Autodesk Fusion 360 part; units mm, degrees
sketch "Sketch1" plane through (0, 0, 0) normal (0, 0, 1) x (1, 0, 0)
  circle A0 centre (0, 0) radius 10.1
  dimension "d1" = 20.2
extrude "Extrude1" add sketch "Sketch1" along normal blind 13.95
sketch "Sketch2" plane through (0, 0, 13.95) normal (0, 0, 1) x (-1, 0, 0)
  circle A0 centre (0, 0) radius 10.1
  circle A1 centre (0, 0) radius 17.5
  line L0 (-27.5, -17.6099) -> (27.5, -17.6099)
  line L1 (27.5, -17.6099) -> (27.5, 17.6099)
  line L2 (27.5, 17.6099) -> (-27.5, 17.6099)
  line L3 (-27.5, 17.6099) -> (-27.5, -17.6099)
  line L4 (-27.5, -17.6099) -> (27.5, 17.6099) construction
  line L5 (27.5, -17.6099) -> (-27.5, 17.6099) construction
  line L6 (-27.5, -17.6099) -> (-42.678, -17.6099)
  line L7 (-42.678, -17.6099) -> (-42.678, 17.6539)
  line L8 (-42.678, 17.6539) -> (-27.5, 17.6539)
  line L9 (-27.5, 17.6539) -> (-27.5, -17.6099)
  dimension "d4" = 35
  dimension "d7" = 55
extrude "Extrude2" add sketch "Sketch2" along normal blind 2 contours A0 | A1
extrude "Extrude3" add sketch "Sketch2" along normal blind 2 contours L0 L1 L2 L3 L9
sketch "Sketch3" plane through (0, 0, 13.95) normal (0, 0, 1) x (-1, 0, 0)
  circle A0 centre (11.0543, 10.2607) radius 1.5
  dimension "d10" = 3
extrude "Extrude4" add sketch "Sketch2" along normal blind 2 contours L3 L6 L7 L8 L9
sketch "Sketch5" plane through (0, -17.6099, 0) normal (0, -1, 0) x (1, 0, 0)
  line L0 (-27.5, 13.95) -> (27.5, 13.95)
  line L1 (27.5, 13.95) -> (27.5, 15.95)
  line L2 (27.5, 15.95) -> (-27.5, 15.95)
  line L3 (-27.5, 15.95) -> (-27.5, 13.95)
  line L4 (-27.5, 15.95) -> (42.6781, 15.95)
  line L5 (42.6781, 15.95) -> (42.6781, 13.95)
  line L6 (42.6781, 13.95) -> (-27.5, 13.95)
  line L7 (-27.5, 13.95) -> (-27.5, 15.95)
extrude "Extrude5" add sketch "Sketch5" along normal blind 35.8
sketch "Sketch6" plane through (42.678, 0, 0) normal (1, 0, 0) x (0, 1, 0)
  line L0 (-17.6099, 15.95) -> (-17.6099, 13.95)
  line L1 (-17.6099, 13.95) -> (17.6099, 13.95)
  line L2 (17.6099, 13.95) -> (17.6099, 15.95)
  line L3 (17.6099, 15.95) -> (-17.6099, 15.95)
  line L4 (17.6099, 15.95) -> (-53.4009, 15.95)
  line L5 (-53.4009, 15.95) -> (-53.4009, 13.9526)
  line L6 (-53.4009, 13.9526) -> (17.6099, 13.9526)
  line L7 (17.6099, 13.9526) -> (17.6099, 15.95)
extrude "Extrude6" add sketch "Sketch6" along normal blind 18 contours L0 L2 L3 L4 L6 L7 | L0 L4 L5 L6
sketch "Sketch7" plane through (-27.5, 0, 0) normal (-1, 0, 0) x (0, -1, 0)
  line L0 (-17.6099, 13.95) -> (53.4099, 13.95)
  line L1 (53.4099, 13.95) -> (53.4099, 15.95)
  line L2 (53.4099, 15.95) -> (-17.6099, 15.95)
  line L3 (-17.6099, 15.95) -> (-17.6099, 13.95)
  line L4 (-17.6099, 15.95) -> (53.4099, 15.95)
  line L5 (53.4099, 15.95) -> (53.4099, 13.95)
  line L6 (53.4099, 13.95) -> (-17.6099, 13.95)
  line L7 (-17.6099, 13.95) -> (-17.6099, 15.95)
extrude "Extrude7" cut sketch "Sketch7" against normal blind 15
sketch "Sketch8" plane through (0, 0, 13.95) normal (0, 0, 1) x (-1, 0, 0)
  circle A0 centre (0, 0) radius 12.0416
extrude "Extrude8" add sketch "Sketch8" against normal blind 2
extrude "Extrude9" add 1 faces at (30.2854, -6.0604, 15.95) along direction (0, 0, 1) blind 1
Can you work these out from the model? Positions are in its coordinate system, mm. A direction names the side the tool comes from. Round coordinates to 2 decimals unless told otherwise and drop trailing zeros. Order: outer loops, then holes, each group sorted by start corner. A loop starts at its lowest first (then second) coordinate and runs counter-clockwise, first axis right, second up. Notation, with made-up numbers: (32.25, -28) -> (44.25, -28) arc R21 ccw to (44.25, 6) -> close; hole circle Ø3 at (49.5, 65.25). An arc over 180 degrees is marked (long way). Write each question's results on one line, items separated by ' | '. Start each with the question number.
Item 1: Will these pins go through, and if not, where does the flat tip stop? pin 1 (14.5 mm diameter, centred on x = 48, y = -1, fed in from -Z); pin 2 (3.5 mm diameter, centred on x = 53.5, z = 15, fed in from -Y).
Item 2: If we section it at B-B, the plane x = 0: Write out the boundary of the cut face in (y, z), then the cut area to 3 significant figures.
Item 3: Please list where these lines run through material, in increasing order: L1, parallel to Z at x = 23, y = -7.5; L2, parallel to Y at x = -0.5, z = 9.5; L3, parallel to X at y = 6.5, z = 6.25.
Item 4: Which directions (+Z, -Z, +X, -X, +Y, -Y) give clear straight access to the entire face, cutting with the end or side of a thin tool? Please do faces 1 (the flat face through (60.678, -18, 15)), 2 (the flat face through (-3, 10, 11.95)), 3 (the flat face through (52, -18, 13.953)).
Item 5: If we section it at D-D, the plane z = 8.25: Write out the boundary of the cut face in (x, y).
Results:
1) pin 1: stops at z = 13.95 | pin 2: stops at y = -53.4
2) outline: (-53.41, 13.95) -> (-12.04, 13.95) -> (-12.04, 11.95) -> (-10.1, 11.95) -> (-10.1, 0) -> (10.1, 0) -> (10.1, 11.95) -> (12.04, 11.95) -> (12.04, 13.95) -> (17.61, 13.95) -> (17.61, 16.95) -> (-53.41, 16.95) -> close | area: 503 mm2
3) L1: z = 13.95 to 16.95 | L2: y = -10.09 to 10.09 | L3: x = -7.73 to 7.73
4) face 1: +Z, -Z, +X, +Y, -Y | face 2: -Z | face 3: -Z, +X, +Y, -Y
5) outline: circle Ø20.2 at (0, 0)
